Part model, mm, in its own coordinate system. A direction names the side the tool comes from. Give positions to 0.01 mm unless a question says otherwise; leave off trailing zeros. Write each loop counter-clockwise with the first axis right and the second up, starting at its lowest first coordinate (ties: lowest second). Pieces come first, ordered by that corner, then holes. Notation, with made-up numbers: M 42.5,70.5 L 52.5,70.5 A22 ccw 52.5,101.5 Z; hole C 3.5,20.5 d9. An arc over 180 degrees is marked long. Use CSV: the item, a comma, the result in double quotes. Start each with the question number.
1. Band-saw the part on D-D, the plane z = 14.75. List the corners of the cut face in (x, y).
2. Drill centre lines: line 1 along X through (y, z) = (-0.75, 9.25); line 2 along Z through (x, y) = (0.6, -6.35). Where is each one in solid material? Low to high. Write a range as from..to.
3. Drop flat-ended pins along their axis: pin 1 Ø4 at (y, z) = (-6.35, 20.74) entering from +X; pin 2 Ø4 at (y, z) = (-7.5, 16.5) entering from +X; pin 3 Ø1.5 at (x, y) = (8.5, -2.5) entering from +Z. Give the stop position or say it passes through.
4. Band-saw the part on C-C, the plane y = -11. List the corners of the cut face in (x, z) (3 decimals), then the cut area to 3 significant figures.
5. Mould opens along Y. For faces 1 (the face through (0, -6, 14)), 2 (the face through (23.669, -7.566, 0.811)), 3 (the face through (1, 0, 7)) say: pulls with the +Y half, pulls with the -Y half, needs draft (parallel to the pull), parting line crosses it, or undercut.
6. Band-saw the part on A-A, the plane y = -6.35. List the corners of the cut face in (x, z) (3 decimals).
7. Band-saw the part on B-B, the plane x = 19. List the corners of the cut face in (y, z).
8. 3-axis set-ups, long thin cutter, end or side, ignore diameter. For faces 4 (the face through (15, -6, 1.6)), 5 (the face through (1, -12.7, 7)): which of +Z, -Z, +X, -X, +Y, -Y reach the whole face in a straight line?
from build123d import *

# Parameters (mm, degrees)
F1_DEPTH = 12.7
F2_R     = 3.175
F3_DEPTH = 25.4
F4_R     = 3.175
F5_DEPTH = 25.4


with BuildPart() as f1:
    # F0 (on Front) → F1 (new body)
    with BuildSketch(Plane.XZ):
        with BuildLine():
            Line((0, 25.4), (0, 3.175))
            ThreePointArc((0, 3.175), (0.929936, 0.929936), (3.175, 0))
            Line((3.175, 0), (25.4, 0))
            Line((25.4, 0), (25.4, 1.6002))
            Line((25.4, 1.6002), (4.7752, 1.6002))
            ThreePointArc((4.7752, 1.6002), (2.530136, 2.530136), (1.6002, 4.7752))
            Line((1.6002, 4.7752), (1.6002, 25.4))
            Line((1.6002, 25.4), (0, 25.4))
        make_face()
    extrude(amount=F1_DEPTH)

    # F2 (on face) → F3 (cut)
    with BuildSketch(Plane.XY.offset(1.6002)):
        with Locations((20.73656, -6.35)):
            Circle(F2_R)
    extrude(amount=-F3_DEPTH, mode=Mode.SUBTRACT)

    # F4 (on face) → F5 (cut)
    with BuildSketch(Plane.YZ.offset(1.6002)):
        with Locations((-6.35, 20.73656)):
            Circle(F4_R)
    extrude(amount=-F5_DEPTH, mode=Mode.SUBTRACT)


solid = f1.part
Output:
1,outline,"M 0,-12.7 L 1.6,-12.7 L 1.6,0 L 0,0 Z"
2,line 1,"x = 0..1.6"
2,line 2,"z = 1.32..17.56, 23.91..25.4"
3,pin 1,"passes through"
3,pin 2,"stops at x = 1.6"
3,pin 3,"stops at z = 1.6"
4,outline,"M 0,3.175 A3.175 ccw 3.175,0 L 25.4,0 L 25.4,1.6 L 4.775,1.6 A3.175 cw 1.6,4.775 L 1.6,25.4 L 0,25.4 Z"
4,area,"78.7 mm²"
5,face 1,"needs draft"
5,face 2,"undercut"
5,face 3,"pulls with the +Y half"
6,outline,"M 0,3.175 A3.175 ccw 3.175,0 L 17.562,0 L 17.562,1.6 L 4.775,1.6 A3.175 cw 1.6,4.775 L 1.6,17.562 L 0,17.562 Z; M 0,23.912 L 1.6,23.912 L 1.6,25.4 L 0,25.4 Z; M 23.912,0 L 25.4,0 L 25.4,1.6 L 23.912,1.6 Z"
7,outline,"M -12.7,0 L -9.01,0 L -9.01,1.6 L -12.7,1.6 Z; M -3.69,0 L 0,0 L 0,1.6 L -3.69,1.6 Z"
8,face 4,"+Z, +X, +Y, -Y"
8,face 5,"+Z, -Z, +X, -X, -Y"
